Design review of the part shown in the three views and the two pictorial views. Dimensions are in mm from the part's minimum x, y and z. A direction names the side the tool comes from. Coordinates: 2 decimals unless noted, no trailing zeros. Loops run counter-clockwise (first coordinate to the right, second up) from the corner with the lowest first, then second, coordinate; pieces in that order, holes last. Notation, with made-up numbers: M 15.25,-3 L 70.25,-3 A21 ccw 70.25,24 Z; hole C 67,47 d4. An arc over 180 degrees is marked long. Write item = value, one per line. Start each with the question number.
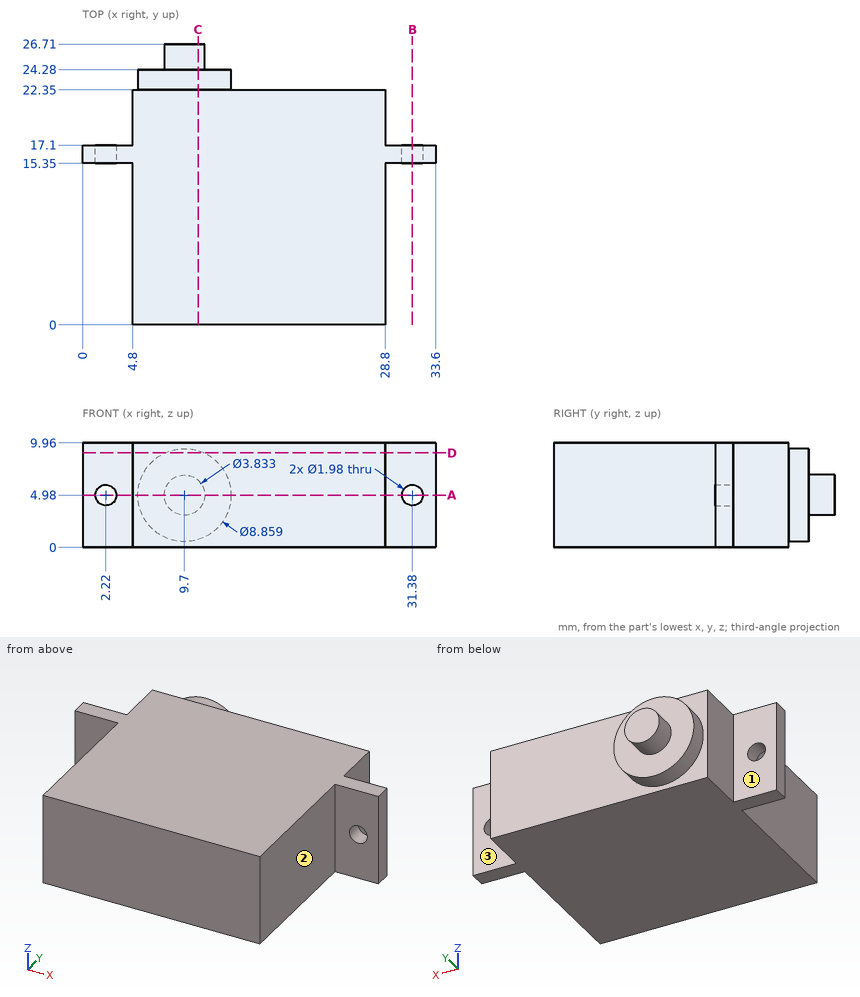
(1) Take a section at A-A (z = 4.98). State the section outline as (x, y) points, plus the area to 3 significant figures.
(2) To check wall thickness, follow L1, parallel to X at y = 16.7, z = 4.98; L2, parallel to Z at x = 31.38, y = 16.7; L3, parallel to X at y = 2.25, z = 2.25. State the ranges of each line that lie inside material, in increasing order.
(3) Take a section at B-B (x = 31.38). State the section outline as (y, z) points, plus the area to 3 significant figures.
(4) Tool access review of the marked faces 1, 2 and 3: name each direction out of +Z, -Z, +X, -X, +Y, -Y from which nothing blocks a thin tool from reaching the whole face with its end or side.
(5) Take a section at D-D (z = 9). State the section outline as (x, y) points.
(6) Take a section at C-C (x = 11). State the section outline as (y, z) points.
(7) Insertion check: pin 1 (4 mm diameter, centred on x = 31.5, z = 6.5, fed in from +Y); pin 2 (3 mm diameter, centred on y = 7.5, z = 2.5, fed in from -X); pin 3 (1.4 mm diameter, centred on x = 32.5, z = 3, fed in from -Y); pin 4 (4 mm diameter, centred on x = 28.5, z = 1.5, fed in from -Y). Each pin has a flat end and moves straight along its axis. Give the tip position at first contact, or say it passes through.
Results list:
q1.outline = M 0,15.35 L 1.23,15.35 L 1.23,17.1 L 0,17.1 Z; M 3.21,15.35 L 4.8,15.35 L 4.8,0 L 28.8,0 L 28.8,15.35 L 30.39,15.35 L 30.39,17.1 L 28.8,17.1 L 28.8,22.35 L 14.13,22.35 L 14.13,24.28 L 11.62,24.28 L 11.62,26.71 L 7.78,26.71 L 7.78,24.28 L 5.27,24.28 L 5.27,22.35 L 4.8,22.35 L 4.8,17.1 L 3.21,17.1 Z; M 32.37,15.35 L 33.6,15.35 L 33.6,17.1 L 32.37,17.1 Z
q1.area = 573 mm^2
q2.L1 = 0 to 1.23, 3.21 to 30.39, 32.37 to 33.6
q2.L2 = 0 to 3.99, 5.97 to 9.96
q2.L3 = 4.8 to 28.8
q3.outline = M 15.35,0 L 17.1,0 L 17.1,3.99 L 15.35,3.99 Z; M 15.35,5.97 L 17.1,5.97 L 17.1,9.96 L 15.35,9.96 Z
q3.area = 14.0 mm^2
q4.face_1 = +Z, -Z, -X, +Y
q4.face_2 = +Z, -Z, +X, -Y
q4.face_3 = +Z, -Z, +X, +Y
q5.outline = M 0,15.35 L 4.8,15.35 L 4.8,0 L 28.8,0 L 28.8,15.35 L 33.6,15.35 L 33.6,17.1 L 28.8,17.1 L 28.8,22.35 L 11.56,22.35 L 11.56,24.28 L 7.84,24.28 L 7.84,22.35 L 4.8,22.35 L 4.8,17.1 L 0,17.1 Z
q6.outline = M 0,0 L 22.35,0 L 22.35,0.75 L 24.28,0.75 L 24.28,3.57 L 26.71,3.57 L 26.71,6.39 L 24.28,6.39 L 24.28,9.21 L 22.35,9.21 L 22.35,9.96 L 0,9.96 Z
q7.pin_1 = 17.1
q7.pin_2 = 4.8
q7.pin_3 = 15.35
q7.pin_4 = 0
